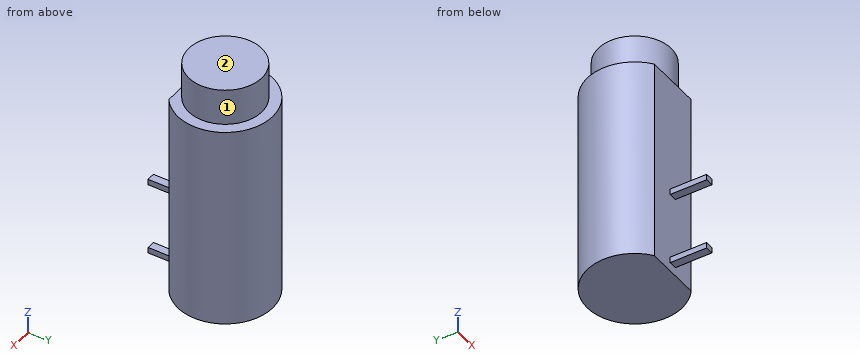
```python
from build123d import *

# Parameters (mm, degrees)
EXTRUDE_1_DEPTH     = 33.1
CUT_EXTRUDE_START   = -5
SKETCH_2_R          = 5
CUT_EXTRUDE_1_DEPTH = 5
SKETCH_3_W          = 1.1
SKETCH_3_H          = 0.8
EXTRUDE_2_DEPTH     = 5


with BuildPart() as part:
    # 草图1 → 凸台-拉伸1 (new body)
    with BuildSketch(Plane.XY):
        with BuildLine():
            Line((-3.9, -5.2), (3.9, -5.2))
            ThreePointArc((3.9, -5.2), (0, 6.5), (-3.9, -5.2))
        make_face()
    extrude(amount=EXTRUDE_1_DEPTH)

    # 草图2 → 切除-拉伸1 (cut)
    with BuildSketch(Plane.XY.offset(33.1).offset(CUT_EXTRUDE_START)):
        with BuildLine():
            Line((-3.9, -5.2), (3.9, -5.2))
            ThreePointArc((3.9, -5.2), (0, 6.5), (-3.9, -5.2))
        make_face()
        Circle(SKETCH_2_R, mode=Mode.SUBTRACT)
    extrude(amount=CUT_EXTRUDE_1_DEPTH, mode=Mode.SUBTRACT)

    # 草图3 → 凸台-拉伸2 (add)
    with BuildSketch(Plane.XZ.offset(5.2)):
        with Locations((0, 11.6)):
            Rectangle(SKETCH_3_W, SKETCH_3_H)
        with Locations((0, 1.6)):
            Rectangle(SKETCH_3_W, SKETCH_3_H)
    extrude(amount=EXTRUDE_2_DEPTH)


solid = part.part
```
Model file for the job. Use its own axes, mm. Face numbers are marked on the shaded views. A direction names the side the tool comes from. Coordinates: 2 decimals unless noted, no trailing zeros. Loops run counter-clockwise (first coordinate to the right, second up) from the corner with the lowest first, then second, coordinate; pieces in that order, holes last. Notation, with made-up numbers: M 19.5,51 L 72.5,51 A19 ccw 72.5,84 Z; hole C -26,42.5 d1. An arc over 180 degrees is marked long. Use CSV: the item, a comma, the result in double quotes. Start each with the question number.
1. Probe probe 1 along Z at (x, y) = (0, -9.5); probe 2 along Z at (x, y) = (-1.75, -4.75); probe 3 along Y at (x, z) = (4.25, 19). List the from-to ranges inside material, lowest first. Write a range as [from, to].
2. Band-saw the part on B-B, the plane y = 0. List the corners of the cut face in (x, z).
3. Band-saw the part on C-C, the plane x = 0. List the corners of the cut face in (y, z).
4. Flat gauge pins, fed straight in: pin 1 (0.6 mm diameter, centred on x = 0, y = -8, fed in from -Z); pin 2 (0.9 mm diameter, centred on y = -7.5, z = 11.5, fed in from -X); pin 3 (0.9 mm diameter, centred on y = -9, z = 11.5, fed in from +X). Where does each tip first touch, or does it go through?
5. Band-saw the part on D-D, the plane z = 19. List the corners of the cut face in (x, y).
6. Tool access for the marked faces 1 and 2: list every direction of +Z, -Z, +X, -X, +Y, -Y with a clear straight run to the whole face (end or side of a thin tool).
7. Band-saw the part on A-A, the plane y = -9. List the corners of the cut face in (x, z), then the cut area to 3 significant figures.
Entries:
1,probe 1,"z = [1.2, 2], [11.2, 12]"
1,probe 2,"z = [0, 28.1]"
1,probe 3,"y = [-4.92, 4.92]"
2,outline,"M -6.5,0 L 6.5,0 L 6.5,28.1 L 5,28.1 L 5,33.1 L -5,33.1 L -5,28.1 L -6.5,28.1 Z"
3,outline,"M -10.2,1.2 L -5.2,1.2 L -5.2,0 L 6.5,0 L 6.5,28.1 L 5,28.1 L 5,33.1 L -5,33.1 L -5,28.1 L -5.2,28.1 L -5.2,12 L -10.2,12 L -10.2,11.2 L -5.2,11.2 L -5.2,2 L -10.2,2 Z"
4,pin 1,"stops at z = 1.2"
4,pin 2,"stops at x = -0.55"
4,pin 3,"stops at x = 0.55"
5,outline,"M -3.9,-5.2 L 3.9,-5.2 A6.5 ccw long Z"
6,face 1,"+Z"
6,face 2,"+Z, +X, -X, +Y, -Y"
7,outline,"M -0.55,1.2 L 0.55,1.2 L 0.55,2 L -0.55,2 Z; M -0.55,11.2 L 0.55,11.2 L 0.55,12 L -0.55,12 Z"
7,area,"1.76 mm2"
